```python
from build123d import *

# Parameters (mm, degrees)
F0_W     = 200
F0_H     = 15
F0_R     = 2.6
F0_R_2   = 1.85
F0_R_3   = 1.5
F1_DEPTH = 10
F2_SIZE  = 2
F3_R     = 1.5
F4_DEPTH = 10
F5_R     = 1.5
F6_DEPTH = 10


with BuildPart() as f1:
    # F0 (on Top) → F1 (new body)
    with BuildSketch(Plane.XY):
        Rectangle(F0_W, F0_H)
        with Locations((-88, 0)):
            Circle(F0_R, mode=Mode.SUBTRACT)
        with Locations((-66.45, 0)):
            Circle(F0_R_2, mode=Mode.SUBTRACT)
        with Locations((-35, 0)):
            Circle(F0_R_3, mode=Mode.SUBTRACT)
        with Locations((-15, 0)):
            Circle(F0_R_3, mode=Mode.SUBTRACT)
        with Locations((15, 0)):
            Circle(F0_R_3, mode=Mode.SUBTRACT)
        with Locations((35, 0)):
            Circle(F0_R_3, mode=Mode.SUBTRACT)
        with Locations((66.45, 0)):
            Circle(F0_R_2, mode=Mode.SUBTRACT)
        with Locations((88, 0)):
            Circle(F0_R, mode=Mode.SUBTRACT)
    extrude(amount=F1_DEPTH)

    # F2
    f2_edges = [f1.edges().sort_by_distance(p)[0] for p in [
        (0, 7.5, 10),
        (0, -7.5, 10),
    ]]
    chamfer(f2_edges, length=F2_SIZE)

    # F3 (on face) → F4 (cut)
    with BuildSketch(Plane.YZ.offset(100)):
        with Locations((0, 5)):
            Circle(F3_R)
    extrude(amount=-F4_DEPTH, mode=Mode.SUBTRACT)

    # F5 (on face) → F6 (cut)
    with BuildSketch(Plane(origin=(-100, 0, 0), x_dir=(0, -1, 0), z_dir=(-1, 0, 0))):
        with Locations((0, 5)):
            Circle(F5_R)
    extrude(amount=-F6_DEPTH, mode=Mode.SUBTRACT)


solid = f1.part
```
Geometry check sheet. Reference: the model listing, model coordinates, mm. Give positions to 0.01 mm unless a question says otherwise; leave off trailing zeros. Order: outer loops, then holes, each group sorted by start corner. A loop starts at its lowest first (then second) coordinate and runs counter-clockwise, first axis right, second up.
1. Release check for a two-part mould opening along Y. For faces 1 (the face through (-1, 7.5, 4)), 2 (the face through (-64.74, -0.71, 4.93)), 3 (the face through (-85.52, 0.78, 4.93)), 4 (the face through (100, -2, 5)) record: pulls with the +Y half, pulls with the -Y half, needs draft (parallel to the pull), parting line crosses it, or undercut.
2. Section check A-A, the plane x = 88. Enter the section's corners in (y, z), and give its area (3 significant figures).
3. Thickness scan on L1, parallel to Z at x = -97, y = 0; L2, parallel to Y at x = -15, z = 2.5; L3, parallel to X at y = 2.25, z = 5.75. Record the ranges inside material, lowest first.
4. Section check B-B, the plane x = 66.45. Enter the section's corners in (y, z).
Values follow:
1. face 1: pulls with the +Y half
1. face 2: undercut
1. face 3: undercut
1. face 4: needs draft
2. outline: (-7.5, 0) - (-2.6, 0) - (-2.6, 10) - (-5.5, 10) - (-7.5, 8) - close; (2.6, 0) - (7.5, 0) - (7.5, 8) - (5.5, 10) - (2.6, 10) - close
2. area: 94.0 mm2
3. L1: z = 0 to 3.5, 6.5 to 10
3. L2: y = -7.5 to -1.5, 1.5 to 7.5
3. L3: x = -100 to -89.3, -86.7 to 86.7, 89.3 to 100
4. outline: (-7.5, 0) - (-1.85, 0) - (-1.85, 10) - (-5.5, 10) - (-7.5, 8) - close; (1.85, 0) - (7.5, 0) - (7.5, 8) - (5.5, 10) - (1.85, 10) - close
